from build123d import *

# Parameters (mm, degrees)
SKETCH_1_W          = 40
SKETCH_1_H          = 30
SKETCH_1_W_2        = 38
SKETCH_1_H_2        = 28
EXTRUDE_1_DEPTH     = 175
SKETCH_2_R          = 1.525
CUT_EXTRUDE_1_DEPTH = 10
SKETCH_3_R          = 3.5
CUT_EXTRUDE_2_DEPTH = 10
SKETCH_5_R          = 1.525
CUT_EXTRUDE_3_DEPTH = 10
CUT_EXTRUDE_4_DEPTH = 80
SKETCH_7_R          = 1.55
CUT_EXTRUDE_5_DEPTH = 80


with BuildPart() as part:
    # 草图1 → 凸台-拉伸1 (new, symmetric)
    with BuildSketch(Plane.XY):
        Rectangle(SKETCH_1_W, SKETCH_1_H)
        Rectangle(SKETCH_1_W_2, SKETCH_1_H_2, mode=Mode.SUBTRACT)
    extrude(amount=EXTRUDE_1_DEPTH, both=True)

    # 草图2 → 切除-拉伸1 (cut)
    with BuildSketch(Plane(origin=(20, 0, 0), x_dir=(0, 0, -1), z_dir=(1, 0, 0))):
        with Locations((0, -3)):
            Circle(SKETCH_2_R)
        with Locations((-100, -3)):
            Circle(SKETCH_2_R)
        with Locations(Location((100, -3, 0), (0, 0, 270))):
            Circle(SKETCH_2_R)
    extrude(amount=-CUT_EXTRUDE_1_DEPTH, mode=Mode.SUBTRACT)

    # 草图3 → 切除-拉伸2 (cut)
    with BuildSketch(Plane(origin=(-19, 0, 0), x_dir=(0, 0, -1), z_dir=(1, 0, 0))):
        with Locations((-100, -3)):
            Circle(SKETCH_3_R)
        with Locations((0, -3)):
            Circle(SKETCH_3_R)
        with Locations((100, -3)):
            Circle(SKETCH_3_R)
    extrude(amount=-CUT_EXTRUDE_2_DEPTH, mode=Mode.SUBTRACT)

    # 草图5 → 切除-拉伸3 (cut)
    with BuildSketch(Plane.ZY.offset(20)):
        with Locations((125, -3)):
            Circle(SKETCH_5_R)
        with Locations((-125, -3)):
            Circle(SKETCH_5_R)
        with Locations((-50, -3)):
            Circle(SKETCH_5_R)
        with Locations((50, -3)):
            Circle(SKETCH_5_R)
    extrude(amount=-CUT_EXTRUDE_3_DEPTH, mode=Mode.SUBTRACT)

    # 草图6 → 切除-拉伸4 (cut)
    with BuildSketch(Plane.XZ.offset(15)):
        with BuildLine():
            Line((-8, 120), (-8, 130))
            ThreePointArc((-8, 130), (0, 138), (8, 130))
            Line((8, 130), (8, 120))
            ThreePointArc((8, 120), (0, 112), (-8, 120))
        make_face()
        with BuildLine():
            Line((-8, 45), (-8, 55))
            ThreePointArc((-8, 55), (0, 63), (8, 55))
            Line((8, 55), (8, 45))
            ThreePointArc((8, 45), (0, 37), (-8, 45))
        make_face()
    cut_extrude_4 = extrude(amount=-CUT_EXTRUDE_4_DEPTH, mode=Mode.SUBTRACT)

    # 镜向1: 切除-拉伸4 across plane
    add(cut_extrude_4.mirror(Plane.XY), mode=Mode.SUBTRACT)

    # 草图7 → 切除-拉伸5 (cut)
    with BuildSketch(Plane(origin=(0, 15, 0), x_dir=(1, 0, 0), z_dir=(0, 1, 0))):
        with Locations(Location((16, 171, 0), (0, 0, 180))):
            Circle(SKETCH_7_R)
        with Locations(Location((16, 154, 0), (0, 0, 180))):
            Circle(SKETCH_7_R)
        with Locations(Location((-16, 154, 0), (0, 0, 180))):
            Circle(SKETCH_7_R)
        with Locations(Location((-16, 171, 0), (0, 0, 180))):
            Circle(SKETCH_7_R)
    cut_extrude_5 = extrude(amount=-CUT_EXTRUDE_5_DEPTH, mode=Mode.SUBTRACT)

    # 镜向2: 切除-拉伸5 across plane
    add(cut_extrude_5.mirror(Plane.XY), mode=Mode.SUBTRACT)


solid = part.part
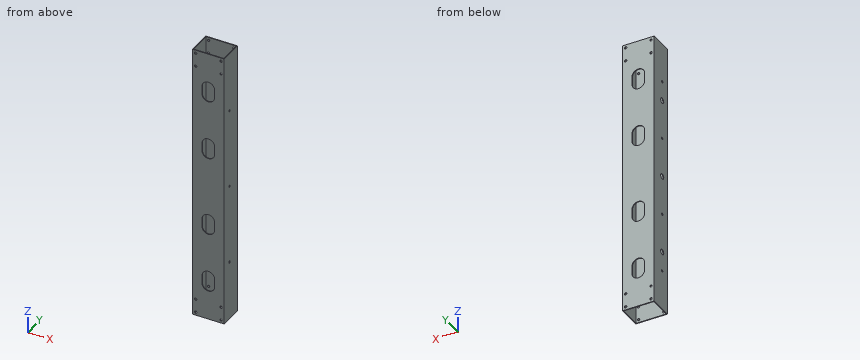
The model under review builds one solid part; all positions refer to its coordinate system, in mm. Coordinates: 2 decimals unless noted, no trailing zeros. Loops run counter-clockwise (first coordinate to the right, second up) from the corner with the lowest first, then second, coordinate; pieces in that order, holes last. Notation, with made-up numbers: M 63,-7 L 75,-7 A18 cw 75,20 Z; hole C 57.5,-16 d8. An arc over 180 degrees is marked long. Put each result on its own line as item: value. Start each with the question number.
Q1. Add section B-B (z = 26). Write out the cut boundary in (x, y).
Q2. Wall thickness on line 1 (Z direction, x = -16, y = 14.8); line 2 (X direction, y = 14.8, z = 171); line 3 (X direction, y = 5, z = -5): over which ranges is each line inside the solid? List them lowest first.
Q3. Add section C-C (x = -11). Write out the cut boundary in (y, z).
Q4. Add section A-A (y = 4.5). Write out the cut boundary in (x, z).
Answers:
1. outline: M -20,-15 L 20,-15 L 20,15 L -20,15 Z; hole M -19,-14 L 19,-14 L 19,14 L -19,14 Z
2. line 1: z = -175 to -172.55, -169.45 to -155.55, -152.45 to 152.45, 155.55 to 169.45, 172.55 to 175
2. line 2: x = -20 to -17.55, -14.45 to 14.45, 17.55 to 20
2. line 3: x = -20 to -19, 19 to 20
3. outline: M -15,-175 L -14,-175 L -14,175 L -15,175 Z; M 14,-175 L 15,-175 L 15,175 L 14,175 Z
4. outline: M -20,-175 L -19,-175 L -19,175 L -20,175 Z; M 19,-175 L 20,-175 L 20,175 L 19,175 Z
